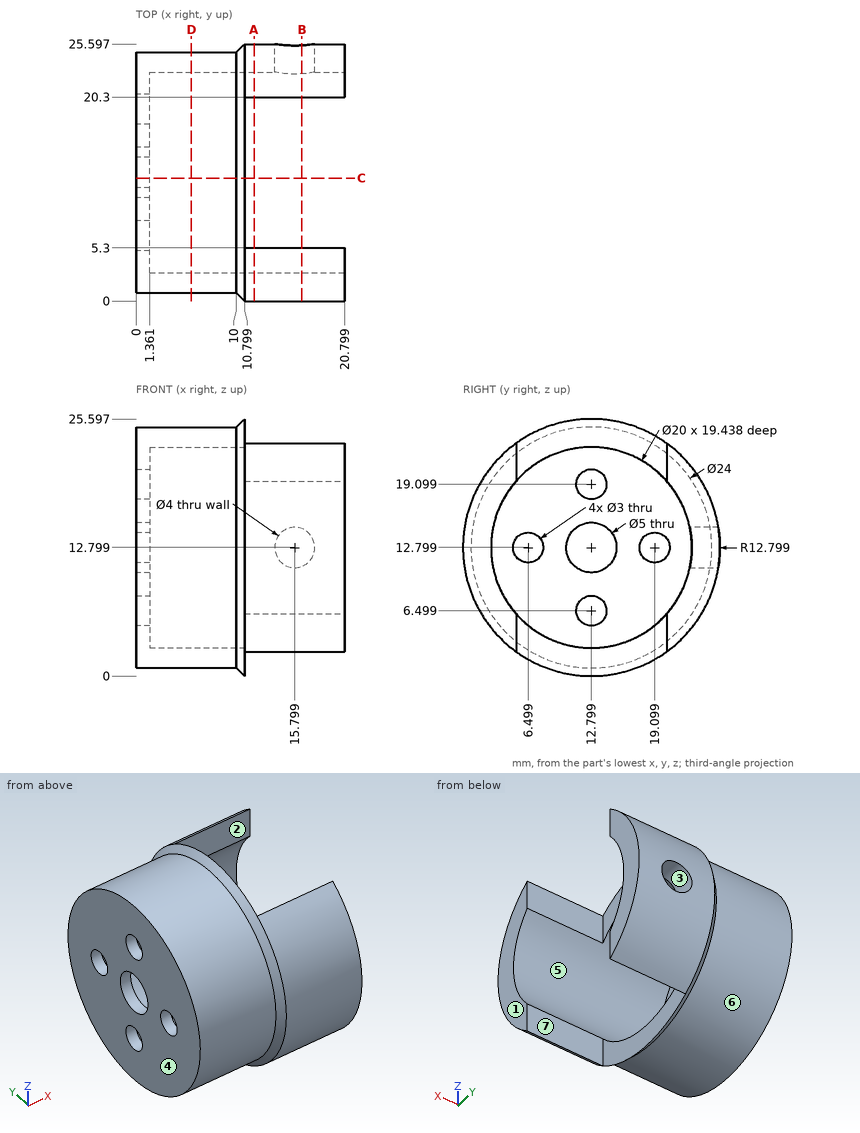
Can you work these out from the drawing? Everything is in mm from the part's minimum corner. A direction names the side the tool comes from. Round coordinates to 2 decimals unless told otherwise and drop trailing zeros. Loops run counter-clockwise (first coordinate to the right, second up) from the corner with the lowest first, then second, coordinate; pieces in that order, holes last. Notation, with made-up numbers: M 57.25,-3.75 L 88.25,-3.75 A9 ccw 88.25,8.25 Z; hole C -14,80 d2. An arc over 180 degrees is marked long. Answer in a Markdown table with one row per item.
1. Please list where these lines run through material, in increasing order: line 1 (Y direction, x = 5.25, z = 12.5) (1 decimal); line 2 (Y direction, x = 18.5, z = 12.75); line 3 (X direction, y = 11.5, z = 17.5). Write a range as from..to.
Established:
| item | result |
|---|---|
| line 1 | 0.8..2.8, 22.8..24.8 |
| line 2 | 0..2.8, 22.8..25.6 |
| line 3 | 0..1.36 |
2. Thinking about a two-plate mould opening in X: for the marked faces 1, 2, 3 and 4, which applies, pulls with the +X half, pulls with the -X half, needs draft (parallel to the pull), parting line crosses it, or undercut?
Established:
| item | result |
|---|---|
| face 1 | pulls with the +X half |
| face 2 | needs draft |
| face 3 | undercut |
| face 4 | pulls with the -X half |
3. If we section it at A-A, the plane x = 11.75: Please give me the cut outline in (y, z) (1 decimal).
Established:
| item | result |
|---|---|
| outline | M 5.3,2.4 L 5.3,6.2 A10 cw 5.3,19.4 L 5.3,23.2 A12.8 ccw Z; M 20.3,2.4 A12.8 ccw 20.3,23.2 L 20.3,19.4 A10 cw 20.3,6.2 Z |
4. If we section it at D-D, the plane x = 5.5: Please give me the cut outline in (y, z).
Established:
| item | result |
|---|---|
| outline | C 12.8,12.8 d24; hole C 12.8,12.8 d20 |
5. If we section it at B-B, the plane x = 16.5: Please give me the cut outline in (y, z) (1 decimal).
Established:
| item | result |
|---|---|
| outline | M 5.3,2.4 L 5.3,6.2 A10 cw 5.3,19.4 L 5.3,23.2 A12.8 ccw Z; M 20.3,2.4 A12.8 ccw 25.5,10.9 L 22.6,10.9 A10 cw 20.3,6.2 Z; M 20.3,19.4 A10 cw 22.6,14.7 L 25.5,14.7 A12.8 ccw 20.3,23.2 Z |
6. I'm going to push flat-ended pins straight in: pin 1 Ø1.5 at (x, y) = (6.5, 22.5) entering from -Z (1 decimal); pin 2 Ø1.9 at (x, z) = (15.5, 21) entering from +Y (1 decimal); pin 3 Ø6 at (x, y) = (16.5, 22.5) entering from -Z. Where does each tip first touch, or does it pass through?
Established:
| item | result |
|---|---|
| pin 1 | z = 4.8 |
| pin 2 | y = 23.3 |
| pin 3 | z = 2.43 |
7. On a 3-axis mill with a long thin cutter (end or side, diameter ignored), from which of +Z, -Z, +X, -X, +Y, -Y can I reach the whole of each face in a straight line? I mean the marked faces 5, 6 and 7. Say none if no direction works.
Established:
| item | result |
|---|---|
| face 5 | +X |
| face 6 | -X |
| face 7 | +Z, -Z, +X |
8. If we section it at C-C, the plane y = 12.25: Give the number of separate pieces and of enclosed holes in the cut face.
Established:
| item | result |
|---|---|
| separate pieces | 4 |
| enclosed holes | 0 |
